```python
from build123d import *

# Parameters (mm, degrees)
SKETCH_1_R      = 3
EXTRUDE_1_DEPTH = 6
SKETCH_2_R      = 18.5
EXTRUDE_2_DEPTH = 6


with BuildPart() as part:
    # 草图1 → 凸台-拉伸1 (new body)
    with BuildSketch(Plane(origin=(0, 0, 0), x_dir=(1, 0, 0), z_dir=(0, 1, 0))):
        with BuildLine():
            Line((-11.489125293, 32), (11.489125293, 32))
            ThreePointArc((11.489125293, 32), (0, -34), (-11.489125293, 32))
        make_face()
        with Locations(Location((0, 27, 0), (0, 0, 270))):
            Circle(SKETCH_1_R, mode=Mode.SUBTRACT)
        with Locations(Location((27, 0, 0), (0, 0, 270))):
            Circle(SKETCH_1_R, mode=Mode.SUBTRACT)
        with Locations(Location((0, -27, 0), (0, 0, 270))):
            Circle(SKETCH_1_R, mode=Mode.SUBTRACT)
        with Locations(Location((-27, 0, 0), (0, 0, 270))):
            Circle(SKETCH_1_R, mode=Mode.SUBTRACT)
    extrude(amount=EXTRUDE_1_DEPTH)

    # 草图2 → 凸台-拉伸2 (add)
    with BuildSketch(Plane(origin=(0, 6, 0), x_dir=(1, 0, 0), z_dir=(0, 1, 0))):
        with Locations(Location((0, 0, 0), (0, 0, 270))):
            Circle(SKETCH_2_R)
    extrude(amount=EXTRUDE_2_DEPTH)

    # 草图3 → 切除-旋转1 (revolve, cut)
    with BuildSketch(Plane.XY, mode=Mode.PRIVATE) as cut_revolve_1_sk:
        Polygon((0, 12), (14.5, 12), (14.5, 6), (8.5, 6), (8.5, 4), (12.5, 4), (12.5, 2), (8.5, 2), (8.5, 0), (0, 0), align=None)
    revolve(cut_revolve_1_sk.sketch.rotate(Axis((0, 0, 0), (0, 1, 0)), 90), axis=Axis((0, 0, 0), (0, 1, 0)), mode=Mode.SUBTRACT)


solid = part.part
```
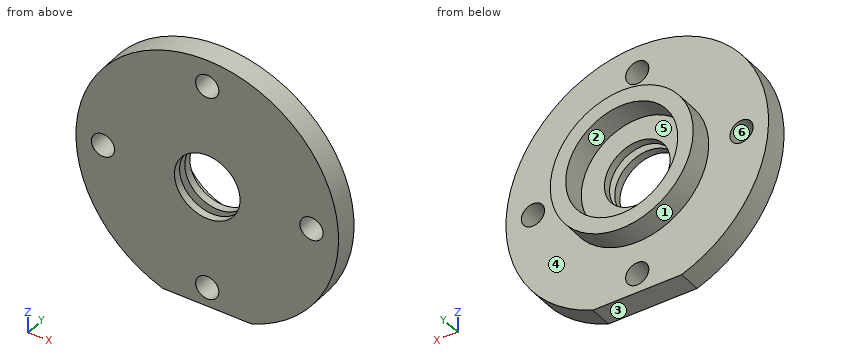
Read the model definition and answer for the solid it produces. Units are mm, in the model's axes. Face numbers are marked on the shaded views. A direction names the side the tool comes from. Round coordinates to 2 decimals unless told otherwise and drop trailing zeros. Write each loop counter-clockwise with the first axis right and the second up, starting at its lowest first coordinate (ties: lowest second). Pieces come first, ordered by that corner, then holes. Notation, with made-up numbers: (-10.75, 15.25) -> (27.25, 15.25) arc R27 ccw to (27.25, 53.25) -> close; hole circle Ø3 at (44, 32). An arc over 180 degrees is marked (long way). Answer in a Markdown table with one row per item. Add a question column.
1) Given P1, Ø1.5, axis at x = 9.5, z = -24, coming from the -Y side; P2, Ø8.5, axis at x = 6.5, z = 2, coming from the +Y side; P3, Ø4, axis at y = 10, z = 4, coming from the -X side, each flat-ended and moving along its own axis, determine where each tip first touches the part or whether it passes through.
2) Find section B-B, the plane y = 1. Determine the outline of the cut face in (x, z), and give its area (3 significant figures).
3) Consider line 1 (X direction, y = 4.25, z = 0); line 2 (Y direction, x = -30.5, z = -1); line 3 (X direction, y = 8.5, z = 7). Determine where each line is inside the solid, lowest interval first.
4) Determine the mould class of the marked faces 1, 2, 3 and 4 for opening direction Z: pulls with the +Z half, pulls with the -Z half, needs draft (parallel to the pull), parting line crosses it, or undercut.
5) Which of the six approach directions +Z, -Z, +X, -X, +Y, -Y give full straight-line access (tool end or side, diameter ignored) to the marked faces 5 and 6?
6) Find section D-D, the plane x = -27. Determine the outline of the cut face in (y, z).
7) Find section A-A, the plane z = 0. State how many separate pieces and enclosed holes the cut face has, and give its area (3 significant figures).
Findings below:
| question | item | result |
|---|---|---|
| 1 | P1 | y = 0 |
| 1 | P2 | y = 6 |
| 1 | P3 | x = -18.39 |
| 2 | outline | (-11.49, -32) -> (11.49, -32) arc R34 ccw (long way) to start; hole circle Ø6 at (-27, 0); hole circle Ø17 at (0, 0); hole circle Ø6 at (0, -27); hole circle Ø6 at (0, 27); hole circle Ø6 at (27, 0) |
| 2 | area | 3,260 mm² |
| 3 | line 1 | -34 to -30, -24 to -8.5, 8.5 to 24, 30 to 34 |
| 3 | line 2 | 0 to 6 |
| 3 | line 3 | -17.12 to -12.7, 12.7 to 17.12 |
| 4 | face 1 | parting line crosses it |
| 4 | face 2 | undercut |
| 4 | face 3 | pulls with the -Z half |
| 4 | face 4 | needs draft |
| 5 | face 5 | +Y |
| 5 | face 6 | +Y, -Y |
| 6 | outline | (0, -20.66) -> (6, -20.66) -> (6, -3) -> (0, -3) -> close; (0, 3) -> (6, 3) -> (6, 20.66) -> (0, 20.66) -> close |
| 7 | separate pieces | 4 |
| 7 | enclosed holes | 0 |
| 7 | area | 266 mm² |
